Design review of the part built by this model. Coordinates are the model's own, in mm. Face numbers are marked on the shaded views. A direction names the side the tool comes from. Give positions to 0.01 mm unless a question says otherwise; leave off trailing zeros. Order: outer loops, then holes, each group sorted by start corner. A loop starts at its lowest first (then second) coordinate and runs counter-clockwise, first axis right, second up. Notation, with made-up numbers: M 55,54.5 L 77,54.5 A11 ccw 77,67.5 Z; hole C 82,-16 d1. An arc over 180 degrees is marked long. Answer as a JSON object with one key per item and string values.
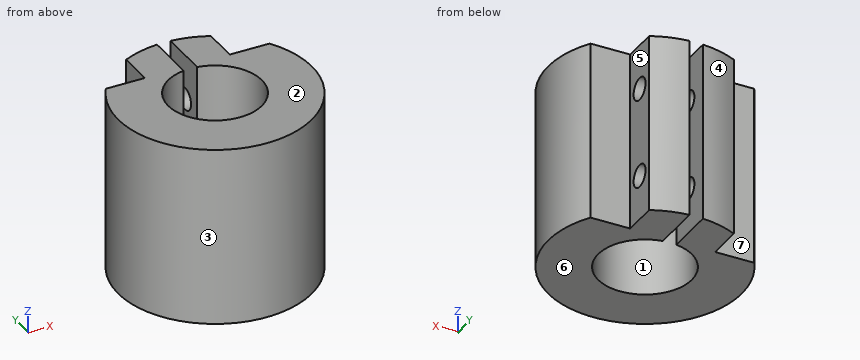
Autodesk Inventor part; units mm, degrees
ref_plane "YZ Plane" through (0, 0, 0) normal (1, 0, 0) x (0, 1, 0)
ref_plane "XZ Plane" through (0, 0, 0) normal (0, 1, 0) x (-1, 0, 0)
ref_plane "XY Plane" through (0, 0, 0) normal (0, 0, 1) x (1, 0, 0)
sketch "Sketch1" plane through (0, 0, 0) normal (0, 0, 1) x (1, 0, 0)
  point P0 (0, 0)
sketch "Sketch2" plane through (0, 0, 0) normal (0, 0, 1) x (1, 0, 0)
  circle A0 centre (0, 0) radius 10.4
  circle A1 centre (0, 0) radius 21.5
  line L0 (0, 10.0548) -> (-1.5, 10.0548)
  line L1 (-1.5, 10.0548) -> (-1.5, 22.3246)
  line L2 (-1.5, 22.3246) -> (1.5, 22.3246)
  line L3 (1.5, 22.3246) -> (1.5, 10.0548)
  line L4 (1.5, 10.0548) -> (0, 10.0548)
  point P0 (1.5, 21.4476)
  point P1 (1.5, 10.2913)
  point P2 (-1.5, 10.2913)
  point P3 (-1.5, 21.4476)
  dimension "d0" = 20.8
  dimension "d1" = 43
  dimension "d3" = 1.5
  dimension "d4" = 3
extrude "Extrusion1" add sketch "Sketch2" along normal blind 40 contours A0 L3 A1 L1 picked at (17.4874, -2.5592)
ref_plane "Work Plane1" through (0, 10.2913, 0) normal (1, 0, 0) x (0, 0, -1)
ref_plane "Work Plane2" through (21.35, 10.2913, 0) normal (1, 0, 0) x (0, 0, -1)
sketch "Sketch3" plane through (21.35, 10.2913, 0) normal (1, 0, 0) x (0, 0, -1)
  line L0 (-40, 0) -> (-40, 11.1564)
  line L1 (-40, 11.1564) -> (-40, 1.1564)
  line L2 (-40, 1.1564) -> (0, 1.1564)
  line L3 (0, 0) -> (-40, 0)
  line L4 (0, 0) -> (0, 11.1564)
  line L5 (0, 1.1564) -> (0, 11.1564)
  line L6 (0, 11.1564) -> (-40, 11.1564)
  line L7 (0, 11.1564) -> (-40, 11.1564)
  point P0 (0, -10.2913)
  dimension "d8" = 10
extrude "Extrusion2" cut sketch "Sketch3" against normal blind 12 contours L0 L6 L4 L2
ref_plane "Work Plane3" through (-21.5, 10.2913, 0) normal (1, 0, 0) x (0, 0, -1)
sketch "Sketch4" plane through (-21.5, 10.2913, 0) normal (1, 0, 0) x (0, 0, -1)
  line L0 (0, 11.1564) -> (-40, 11.1564)
  line L1 (0, 11.1564) -> (0, 1.1564)
  line L2 (0, 11.1564) -> (0, 0)
  line L3 (0, 1.1564) -> (-40, 1.1564)
  line L4 (-40, 0) -> (-40, 11.1564)
  line L5 (-40, 11.1564) -> (0, 11.1564)
  point P0 (0, -10.2913)
  dimension "d12" = 10
extrude "Extrusion3" cut sketch "Sketch4" along normal blind 12
sketch "Sketch5" plane through (9.35, 10.2913, 0) normal (1, 0, 0) x (0, 0, -1)
  circle A0 centre (-30, 5.0692) radius 2.5
  circle A1 centre (-10, 5.0692) radius 2.5
  line L0 (-40, 1.1564) -> (-40, 9.0692)
  line L1 (0, 9.0692) -> (0, 1.1564)
  line L2 (-40, 9.0692) -> (0, 9.0692)
  point P0 (0, -10.2913)
  dimension "d15" = 5
  dimension "d16" = 5
  dimension "d17" = 10
  dimension "d18" = 10
  dimension "d19" = 4
  dimension "d20" = 4
extrude "Extrusion4" cut sketch "Sketch5" against normal through all
properties part number "Cuff"
(1) Insertion check: pin 1 (7 mm diameter, centred on x = -12.5, z = 28.5, fed in from +Y); pin 2 (5 mm diameter, centred on x = -9, z = 24.5, fed in from -Y); pin 3 (6 mm diameter, centred on y = 15.36, z = 30, fed in from -X); pin 4 (3 mm diameter, centred on y = 15.36, z = 30, fed in from +X). Each pin has a flat end and moves straight along its axis. Give the tip position at first contact, or say it passes through.
Checked values:
{"pin 1": "stops at y = 19.53", "pin 2": "stops at y = -20.49", "pin 3": "stops at x = -9.5", "pin 4": "passes through"}
(2) We need section C-C (x = -8). Write out the cut boundary in (y, z).
Checked values:
{"outline": "M -19.96,0 L -6.65,0 L -6.65,40 L -19.96,40 Z; M 6.65,0 L 19.96,0 L 19.96,40 L 6.65,40 Z; hole C 15.36,10 d5; hole C 15.36,30 d5"}
(3) We need section B-B (z = 10). Write out the cut boundary in (x, y).
Checked values:
{"outline": "M -18.2,11.45 A21.5 ccw long 18.2,11.45 L 9.35,11.45 L 9.35,12.86 L 1.5,12.86 L 1.5,10.29 A10.4 cw long -1.5,10.29 L -1.5,12.86 L -9.5,12.86 L -9.5,11.45 Z; M -9.5,17.86 L -1.5,17.86 L -1.5,21.45 A21.5 ccw -9.5,19.29 Z; M 1.5,17.86 L 9.35,17.86 L 9.35,19.36 A21.5 ccw 1.5,21.45 Z"}
(4) Draft analysis for pull direction Y (two halves, no side actions). For the marked faces 1, 2, 3 and 4, state which applies: +Y half, -Y half, draft (parallel to the pull), parting line (faces both ways), or undercut.
Checked values:
{"face 1": "undercut", "face 2": "draft", "face 3": "parting line", "face 4": "+Y half"}
(5) Tool access review of the marked faces 5, 6 and 7: name each direction out of +Z, -Z, +X, -X, +Y, -Y from which nothing blocks a thin tool from reaching the whole face with its end or side.
Checked values:
{"face 5": "+Z, -Z, +X, +Y", "face 6": "-Z, +X, -X, +Y, -Y", "face 7": "+Z, -Z, -X, +Y"}
(6) We need section A-A (y = 0). Write out the cut boundary in (x, z), plus the area to 3 significant figures.
Checked values:
{"outline": "M -21.5,0 L -10.4,0 L -10.4,40 L -21.5,40 Z; M 10.4,0 L 21.5,0 L 21.5,40 L 10.4,40 Z", "area": "888 mm^2"}
(7) We need section D-D (z = 15). Write out the cut boundary in (x, y).
Checked values:
{"outline": "M -18.2,11.45 A21.5 ccw long 18.2,11.45 L 9.35,11.45 L 9.35,19.36 A21.5 ccw 1.5,21.45 L 1.5,10.29 A10.4 cw long -1.5,10.29 L -1.5,21.45 A21.5 ccw -9.5,19.29 L -9.5,11.45 Z"}
(8) To check wall thickness, follow L1, parallel to Z at x = 7.5, y = 15.5; L2, parallel to Y at x = -7.5, z = 30; L3, parallel to X at y = 12, z = 32. State the ranges of each line that lie inside material, in increasing order. Write a range as from..to.
Checked values:
{"L1": "z = 0..7.5, 12.5..27.5, 32.5..40", "L2": "y = -20.15..-7.2, 7.2..12.86, 17.86..20.15", "L3": "x = -9.5..-1.5, 1.5..9.35"}
